from build123d import *
from build123d.topology import SkipClean

# Parameters (mm, degrees)
SKETCH1_R           = 3.5
SKETCH1_R_2         = 21.000776116
SKETCH1_R_3         = 6.35
BOSS_EXTRUDE1_DEPTH = 6.5
SKETCH2_R           = 21.000776116
SKETCH2_R_2         = 17.885901882
BOSS_EXTRUDE2_DEPTH = 6.5
SKETCH3_R           = 10.618204783
SKETCH3_R_2         = 6.35
BOSS_EXTRUDE3_DEPTH = 12.1
SKETCH4_R           = 17.885901882
SKETCH4_R_2         = 10.618204783
BOSS_EXTRUDE5_DEPTH = 4
FILLET1_R           = 6


with BuildPart() as part:
    # Sketch1 → Boss-Extrude1 (new body)
    # profile 1 of 3: a face of its own
    with BuildSketch(Plane(origin=(0, 0, 0), x_dir=(1, 0, 0), z_dir=(0, 1, 0))):
        with BuildLine():
            Line((-33.5, 5), (-33.5, 0))
            Line((-33.5, 0), (-33.5, -5))
            Line((-33.5, -5), (-17.629397896, -11.41213947))
            ThreePointArc((-17.629397896, -11.41213947), (-21.000776116, 0), (-17.629397896, 11.41213947))
            Line((-17.629397896, 11.41213947), (-33.5, 5))
        make_face()
        with Locations(Location((-26.5, 0, 0), (0, 0, 90))):
            Circle(SKETCH1_R, mode=Mode.SUBTRACT)
    # profile 2 of 3: a face of its own
    with BuildSketch(Plane(origin=(0, 0, 0), x_dir=(1, 0, 0), z_dir=(0, 1, 0))):
        Circle(SKETCH1_R_2)
        with Locations(Location((0, 0, 0), (0, 0, 90))):
            Circle(SKETCH1_R_3, mode=Mode.SUBTRACT)
    # profile 3 of 3: a face of its own
    with BuildSketch(Plane(origin=(0, 0, 0), x_dir=(1, 0, 0), z_dir=(0, 1, 0))):
        with BuildLine():
            Line((33.5, 5), (17.629397896, 11.41213947))
            ThreePointArc((17.629397896, 11.41213947), (20.140303321, 5.949855426), (21.000776116, 0))
            ThreePointArc((21.000776116, 0), (20.140303321, -5.949855426), (17.629397896, -11.41213947))
            Line((17.629397896, -11.41213947), (33.5, -5))
            Line((33.5, -5), (33.5, 0))
            Line((33.5, 0), (33.5, 5))
        make_face()
        with Locations(Location((26.5, 0, 0), (0, 0, 90))):
            Circle(SKETCH1_R, mode=Mode.SUBTRACT)
    extrude(amount=BOSS_EXTRUDE1_DEPTH)

    # Sketch2 → Boss-Extrude2 (add)
    with BuildSketch(Plane(origin=(0, 6.5, 0), x_dir=(1, 0, 0), z_dir=(0, 1, 0))):
        with Locations(Location((0, 0, 0), (0, 0, 32.916425521))):
            Circle(SKETCH2_R)
        with Locations(Location((0, 0, 0), (0, 0, 90))):
            Circle(SKETCH2_R_2, mode=Mode.SUBTRACT)
    extrude(amount=BOSS_EXTRUDE2_DEPTH)

    # Sketch3 → Boss-Extrude3 (add)
    with SkipClean():  # the faces are left unmerged after this step: merging them gives an invalid solid
        with BuildSketch(Plane(origin=(0, 6.5, 0), x_dir=(1, 0, 0), z_dir=(0, 1, 0))):
            with Locations(Location((0, 0, 0), (0, 0, 270))):
                Circle(SKETCH3_R)
            with Locations(Location((0, 0, 0), (0, 0, 90))):
                Circle(SKETCH3_R_2, mode=Mode.SUBTRACT)
        extrude(amount=BOSS_EXTRUDE3_DEPTH)

    # Sketch4 → Boss-Extrude5 (add)
    with SkipClean():  # the faces are left unmerged after this step: merging them gives an invalid solid
        with BuildSketch(Plane(origin=(0, 6.5, 0), x_dir=(1, 0, 0), z_dir=(0, 1, 0))):
            with Locations(Location((0, 0, 0), (0, 0, 90))):
                Circle(SKETCH4_R)
            with Locations(Location((0, 0, 0), (0, 0, 270))):
                Circle(SKETCH4_R_2, mode=Mode.SUBTRACT)
        extrude(amount=BOSS_EXTRUDE5_DEPTH)

    # Fillet1
    fillet1_edges = [part.edges().sort_by_distance(p)[0] for p in [
        (33.5, 3.25, 5),
        (33.5, 3.25, -5),
        (-33.5, 3.25, 5),
        (-33.5, 3.25, -5),
    ]]
    fillet(fillet1_edges, radius=FILLET1_R)


solid = part.part
Geometry: final body of the model. Coordinates: model frame, mm. A direction names the side the tool comes from. Coordinates: 2 decimals unless noted, no trailing zeros. Write each loop counter-clockwise with the first axis right and the second up, starting at its lowest first coordinate (ties: lowest second). Pieces come first, ordered by that corner, then holes. Notation, with made-up numbers: (-10, 14) - (32, 14) arc R11 ccw to (32, 35) - close; hole circle Ø5 at (-21.5, 17). An arc over 180 degrees is marked (long way). Return JSON: item names as keys, results as strings.
Item 1: Reachability of faces 1 (the face through (-12.09, 11.73, 13.18)), 2 (the face through (23, 3, 0)) from +Z, -Z, +X, -X, +Y, -Y: full face, straight path, thin tool, end or side. Return the list, or none.
Completed:
{"face 1": "+Y", "face 2": "+Y, -Y"}
Item 2: Pull-direction query (X, two-part tool) for faces 3 (the face through (-8, 0, 0)), 4 (the face through (23.77, 3.2, -8.93)), 5 (the face through (-9.42, 14.49, 4.9)); classes: +X half, -X half, draft (parallel to the pull), parting line (faces both ways), or undercut.
Completed:
{"face 3": "draft", "face 4": "+X half", "face 5": "undercut"}
Item 3: Section query B-B (y = 2.5). Output: boundary loops of the cut face in (x, z), and give its area (3 significant figures).
Completed:
{"outline": "(-33.5, -0.95) arc R6 ccw to (-29.75, -6.52) - (-17.63, -11.41) arc R21 ccw to (17.63, -11.41) - (29.75, -6.52) arc R6 ccw to (33.5, -0.95) - (33.5, 0.95) arc R6 ccw to (29.75, 6.52) - (17.63, 11.41) arc R21 ccw to (-17.63, 11.41) - (-29.75, 6.52) arc R6 ccw to (-33.5, 0.95) - close; hole circle Ø7 at (-26.5, 0); hole circle Ø12.7 at (0, 0); hole circle Ø7 at (26.5, 0)", "area": "1,590 mm2"}
Item 4: Section query A-A (z = 0). Output: boundary loops of the cut face in (x, y), and give its area (3 significant figures).
Completed:
{"outline": "(-33.5, 0) - (-30, 0) - (-30, 6.5) - (-33.5, 6.5) - close; (-23, 0) - (-6.35, 0) - (-6.35, 18.6) - (-10.62, 18.6) - (-10.62, 10.5) - (-17.89, 10.5) - (-17.89, 13) - (-21, 13) - (-21, 6.5) - (-23, 6.5) - close; (6.35, 0) - (23, 0) - (23, 6.5) - (21, 6.5) - (21, 13) - (17.89, 13) - (17.89, 10.5) - (10.62, 10.5) - (10.62, 18.6) - (6.35, 18.6) - close; (30, 0) - (33.5, 0) - (33.5, 6.5) - (30, 6.5) - close", "area": "464 mm2"}
Item 5: Line query: L1, parallel to X at y = 4.5, z = 0; L2, parallel to X at y = 12, z = 0; L3, parallel to X at y = 8.5, z = 0. Output: solid intervals per line, ascending.
Completed:
{"L1": "x = -33.5 to -30, -23 to -6.35, 6.35 to 23, 30 to 33.5", "L2": "x = -21 to -17.89, -10.62 to -6.35, 6.35 to 10.62, 17.89 to 21", "L3": "x = -21 to -6.35, 6.35 to 21"}
Item 6: Section query C-C (x = -24.5). Output: boundary loops of the cut face in (y, z).
Completed:
{"outline": "(0, -8.64) - (6.5, -8.64) - (6.5, -2.87) - (0, -2.87) - close; (0, 2.87) - (6.5, 2.87) - (6.5, 8.64) - (0, 8.64) - close"}
Item 7: Pin query (flat end, axial travel): pin 1 Ø10 at (y, z) = (13, 4) entering from -X; pin 2 Ø8 at (x, z) = (-20, 1.5) entering from +Y; pin 3 Ø10 at (y, z) = (12, -7.5) entering from +X; pin 4 Ø4 at (x, z) = (26.5, 0) entering from +Y. Return the tip coordinate at first contact, or that it passes through.
Completed:
{"pin 1": "stops at x = -21", "pin 2": "stops at y = 13", "pin 3": "stops at x = 20.85", "pin 4": "passes through"}
Item 8: Section query D-D (z = 13). Output: boundary loops of the cut face in (x, y), and give its area (3 significant figures).
Completed:
{"outline": "(-16.49, 0) - (16.49, 0) - (16.49, 13) - (12.28, 13) - (12.28, 10.5) - (-12.28, 10.5) - (-12.28, 13) - (-16.49, 13) - close", "area": "367 mm2"}
